Design review of the part built by this model. Coordinates are the model's own, in mm. Coordinates: 2 decimals unless noted, no trailing zeros. Loops run counter-clockwise (first coordinate to the right, second up) from the corner with the lowest first, then second, coordinate; pieces in that order, holes last. Notation, with made-up numbers: (40, 1.25) -> (88, 1.25) arc R26 ccw to (88, 16.25) -> close; hole circle Ø5 at (86, -35). An arc over 180 degrees is marked (long way). Use a Markdown table: item, result. Add a question column.
Q1. Clearance check with flat-ended pins moving along their axes: pin 1 Ø8 at (y, z) = (732.5, -5) entering from +X; pin 2 Ø2.5 at (x, z) = (0, 0) entering from -Y; pin 3 Ø0.8 at (x, y) = (5.5, 1047.5) entering from -Z; pin 4 Ø1.3 at (x, y) = (6, 1047) entering from +Z. State where each tip first meets the part, or that it passes through.
Q2. Take a section at A-A on y = 388. Write out the cut boundary in (x, z), plus the area to 3 significant figures.
Q3. For probe 1 along Y at (x, z) = (0, -3); probe 2 along Z at (x, y) = (1.35, 4); probe 3 along Y at (x, z) = (-0.5, 1), list the stretches that pass through material, from the lowest coordinate up.
from build123d import *

# Parameters (mm, degrees)
SKETCH1_R           = 5
BOSS_EXTRUDE1_DEPTH = 1050
SKETCH2_R           = 7.5
BOSS_EXTRUDE2_DEPTH = 2
BOSS_EXTRUDE4_DEPTH = 10
SKETCH8_R           = 1
CUT_EXTRUDE1_DEPTH  = 3
SKETCH9_R           = 1
CUT_EXTRUDE2_DEPTH  = 10
CIRPATTERN1_COUNT   = 4


with BuildPart() as part:
    # Sketch1 → Boss-Extrude1 (new body)
    with BuildSketch(Plane(origin=(0, 0, 0), x_dir=(1, 0, 0), z_dir=(0, 1, 0))):
        with Locations(Location((0, 0, 0), (0, 0, 270))):
            Circle(SKETCH1_R)
    extrude(amount=BOSS_EXTRUDE1_DEPTH)

    # Sketch2 → Boss-Extrude2 (add)
    with BuildSketch(Plane(origin=(0, 1040, 0), x_dir=(1, 0, 0), z_dir=(0, 1, 0))):
        with Locations(Location((0, 0, 0), (0, 0, 270))):
            Circle(SKETCH2_R)
    extrude(amount=-BOSS_EXTRUDE2_DEPTH)

    # Sketch4 → Boss-Extrude4 (add)
    with BuildSketch(Plane(origin=(0, 1040, 0), x_dir=(1, 0, 0), z_dir=(0, 1, 0))):
        with BuildLine():
            ThreePointArc((4.898979486, 1), (4.974680765, 0.50254481), (5, 0))
            Line((5, 0), (7.5, 0))
            ThreePointArc((7.5, 0), (7.483239867, 0.501119845), (7.433034374, 1))
            Line((7.433034374, 1), (4.898979486, 1))
        make_face()
        with BuildLine():
            Line((7.5, 0), (5, 0))
            ThreePointArc((5, 0), (4.974680765, -0.50254481), (4.898979486, -1))
            Line((4.898979486, -1), (7.433034374, -1))
            ThreePointArc((7.433034374, -1), (7.483239867, -0.501119845), (7.5, 0))
        make_face()
    extrude(amount=BOSS_EXTRUDE4_DEPTH)

    # Sketch8 → Cut-Extrude1 (cut)
    with BuildSketch(Plane(origin=(0, 1050, 0), x_dir=(1, 0, 0), z_dir=(0, 1, 0))):
        with Locations(Location((0, 0, 0), (0, 0, 270))):
            Circle(SKETCH8_R)
    extrude(amount=-CUT_EXTRUDE1_DEPTH, mode=Mode.SUBTRACT)

    # Sketch9 → Cut-Extrude2 (cut)
    with BuildSketch(Plane.XY):
        with Locations((0, 4)):
            Circle(SKETCH9_R)
    cut_extrude2 = extrude(amount=-CUT_EXTRUDE2_DEPTH, mode=Mode.SUBTRACT)

    # CirPattern1: Cut-Extrude2 ×4 about axis
    cirpattern1_axis = Axis((0, 1050, 0), (0, -1, 0))
    for i in range(1, CIRPATTERN1_COUNT):
        add(cut_extrude2.rotate(cirpattern1_axis, i * 360 / CIRPATTERN1_COUNT), mode=Mode.SUBTRACT)


solid = part.part
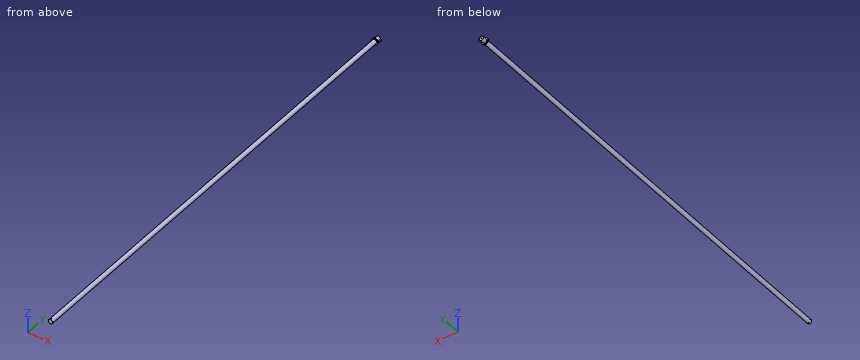
Answer list:
| question | item | result |
|---|---|---|
| 1 | pin 1 | x = 4.9 |
| 1 | pin 2 | y = 0 |
| 1 | pin 3 | z = -1 |
| 1 | pin 4 | z = 1 |
| 2 | outline | circle Ø10 at (0, 0) |
| 2 | area | 78.5 mm² |
| 3 | probe 1 | 0 to 3, 5 to 1050 |
| 3 | probe 2 | -4.81 to -1, 1 to 4.81 |
| 3 | probe 3 | 0 to 3.13, 4.87 to 1050 |
